```python
from build123d import *

# Parameters (mm, degrees)
F1_R     = 16.1
F2_DEPTH = 25.3
F3_R     = 1.575
F4_DEPTH = 2
F5_R     = 2.5
F6_DEPTH = 63
F7_R     = 4
F8_DEPTH = 10


with BuildPart() as f2:
    # F1 (on Front) → F2 (new body)
    with BuildSketch(Plane.XZ):
        with Locations((0, 8.1)):
            Circle(F1_R)
    extrude(amount=-F2_DEPTH)

    # F3 (on Front) → F4 (join)
    with BuildSketch(Plane.XZ):
        with BuildLine():
            ThreePointArc((-19.15, 12.15), (-23.2, 8.1), (-19.15, 4.05))
            Line((-19.15, 4.05), (-15.5822816044, 4.05))
            ThreePointArc((-15.5822816044, 4.05), (-16.1, 8.1), (-15.5822816044, 12.15))
            Line((-15.5822816044, 12.15), (-19.15, 12.15))
        make_face()
        with Locations((-19.15, 8.1)):
            Circle(F3_R, mode=Mode.SUBTRACT)
        with BuildLine():
            Line((19.15, 12.15), (15.5822816044, 12.15))
            ThreePointArc((15.5822816044, 12.15), (16.1, 8.1), (15.5822816044, 4.05))
            Line((15.5822816044, 4.05), (19.15, 4.05))
            ThreePointArc((19.15, 4.05), (23.2, 8.1), (19.15, 12.15))
        make_face()
        with Locations((19.15, 8.1)):
            Circle(F3_R, mode=Mode.SUBTRACT)
    extrude(amount=-F4_DEPTH)

    # F5 (on Front) → F6 (join)
    with BuildSketch(Plane.XZ):
        Circle(F5_R)
    extrude(amount=F6_DEPTH)

    # F7 (on face) → F8 (join)
    with BuildSketch(Plane.XZ):
        Circle(F7_R)
    extrude(amount=F8_DEPTH)


solid = f2.part
```
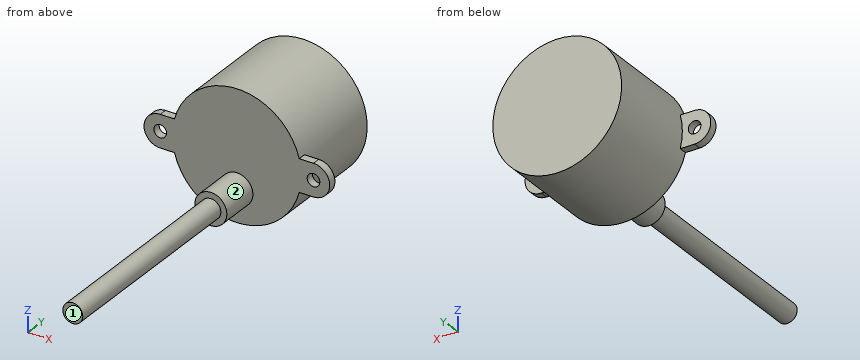
Geometry: final body of the model. Coordinates: model frame, mm. Face numbers are marked on the shaded views. A direction names the side the tool comes from. Round coordinates to 2 decimals unless told otherwise and drop trailing zeros. Order: outer loops, then holes, each group sorted by start corner. A loop starts at its lowest first (then second) coordinate and runs counter-clockwise, first axis right, second up. Notation, with made-up numbers: M -27.5,-22.75 L 8.5,-22.75 A17 cw 8.5,-8.75 Z; hole C 35.25,56 d7. An arc over 180 degrees is marked long. Use one line per item in the form item = value. Start each with the question number.
Q1. Pin query (flat end, axial travel): pin 1 Ø10 at (y, z) = (10, -3) entering from +X; pin 2 Ø10 at (y, z) = (7.5, 8) entering from -X; pin 3 Ø1 at (x, y) = (-17.5, 1.5) entering from +Z. Return the tip coordinate at first contact, or that it passes through.
Q2. Access query for the marked faces 1 and 2. Directions: +Z, -Z, +X, -X, +Y, -Y. A direction counts if a zero-diameter tool reaches every point of the face in a straight line with its end or side. Return the directions, or none.
Q3. Material intervals for line 1 (Z direction, x = 19, y = 1); line 2 (X direction, y = 18.5, z = 8); line 3 (Y direction, x = 6, z = 4), sorted ascending. Write a range as [from, to].
Q4. Cut plane A-A (z = 8.1). Return loops of the section in (x, y) (3 decimals), and give its area (3 significant figures).
Q5. Cut plane B-B (x = 0). Return loops of the section in (y, z).
Q6. Cut plane C-C (z = 0). Return loops of the section in (x, y), and give its area (3 significant figures).
Q7. Cut plane D-D (y = 19.5). Return loops of the section in (x, z), and give its area (3 significant figures).
Geometry results:
q1.pin_1 = 14.9
q1.pin_2 = -16.1
q1.pin_3 = 12.15
q2.face_1 = +Z, -Z, +X, -X, -Y
q2.face_2 = -Y
q3.line_1 = [4.05, 6.53], [9.67, 12.15]
q3.line_2 = [-16.1, 16.1]
q3.line_3 = [0, 25.3]
q4.outline = M -23.2,0 L -20.725,0 L -20.725,2 L -23.2,2 Z; M -17.575,0 L 17.575,0 L 17.575,2 L 16.1,2 L 16.1,25.3 L -16.1,25.3 L -16.1,2 L -17.575,2 Z; M 20.725,0 L 23.2,0 L 23.2,2 L 20.725,2 Z
q4.area = 830 mm^2
q5.outline = M -63,-2.5 L -10,-2.5 L -10,-4 L 0,-4 L 0,-8 L 25.3,-8 L 25.3,24.2 L 0,24.2 L 0,4 L -10,4 L -10,2.5 L -63,2.5 Z
q6.outline = M -13.91,0 L -4,0 L -4,-10 L -2.5,-10 L -2.5,-63 L 2.5,-63 L 2.5,-10 L 4,-10 L 4,0 L 13.91,0 L 13.91,25.3 L -13.91,25.3 Z
q6.area = 1,050 mm^2
q7.outline = C 0,8.1 d32.2
q7.area = 814 mm^2
